For this review, use the dimensioned drawing (mm, ordinates from the lowest corner) and the shaded views. Round coordinates to 2 decimals unless told otherwise and drop trailing zeros. Order: outer loops, then holes, each group sorted by start corner. A loop starts at its lowest first (then second) coordinate and runs counter-clockwise, first axis right, second up. Notation, with made-up numbers: (-21, -10) - (-15, -10) arc R7 ccw to (-15, -6) - close; hole circle Ø9 at (37, 1). An arc over 180 degrees is marked (long way). Write item = value, one per line.
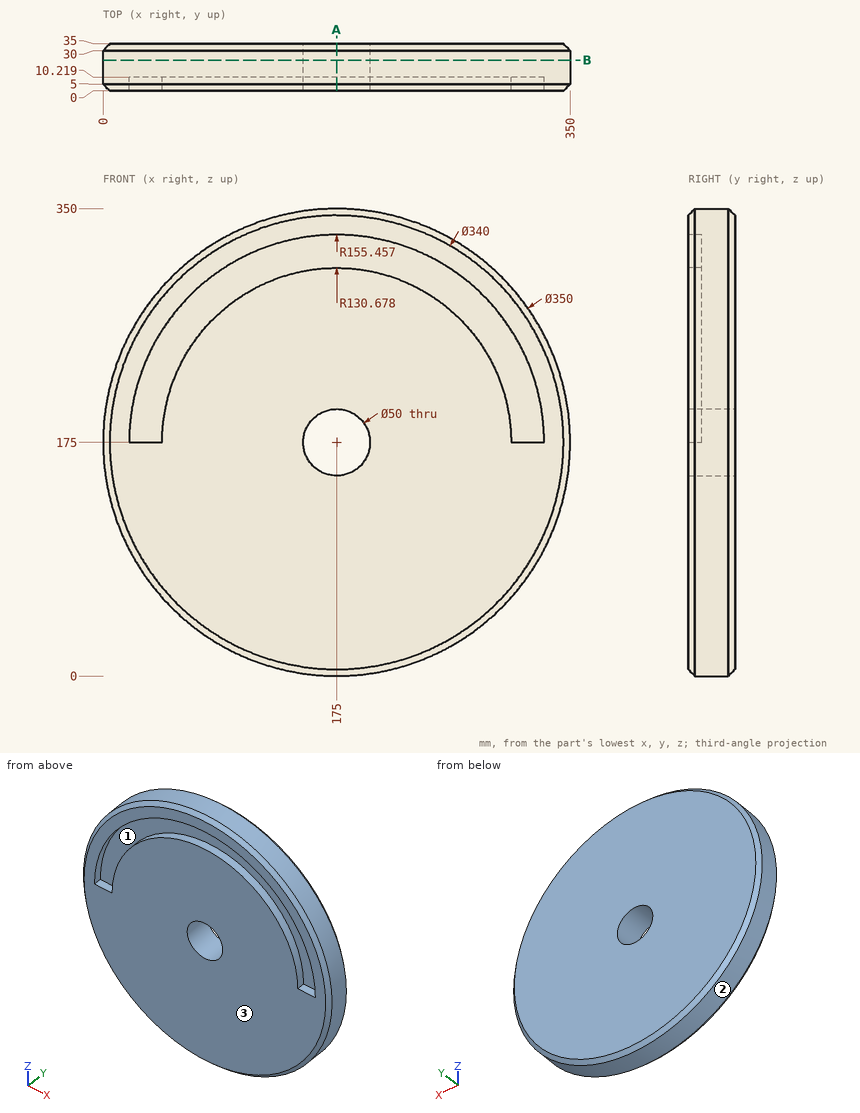
Item 1: Take a section at A-A, the plane x = 175. State the section outline as (y, z) points, and give its area (3 significant figures).
Data:
outline = (0, 5) - (5, 0) - (30, 0) - (35, 5) - (35, 150) - (0, 150) - close; (0, 200) - (35, 200) - (35, 345) - (30, 350) - (5, 350) - (0, 345) - (0, 330.46) - (10.22, 330.46) - (10.22, 305.68) - (0, 305.68) - close
area = 10,200 mm2
Item 2: For line 1 along Z through (x, y) = (175, 10); line 2 along Z through (x, y) = (175, 26); line 3 along Z through (x, y) = (197, 4.5) (1 decimal), list the stretches that pass through material, from the lowest coordinate up. Write a range as [from, to].
Data:
line_1 = [0, 150], [200, 305.68], [330.46, 350]
line_2 = [0, 150], [200, 350]
line_3 = [1.9, 163.1], [186.9, 303.8], [328.9, 348.1]
Item 3: Take a section at B-B, the plane y = 23. State the section outline as (x, z) points, and give its area (3 significant figures).
Data:
outline = circle Ø350 at (175, 175); hole circle Ø50 at (175, 175)
area = 94,200 mm2
Item 4: Insertion check: P1, Ø4, axis at x = 206, y = 14.5, coming from the -Z side; P2, Ø12, axis at y = 18.5, z = 163, coming from the -X side; P3, Ø3, axis at x = 101.5, y = 16, coming from the -Z side. Each pin has a flat end and moves straight along its axis. Give the tip position at first contact, or say it passes through.
Data:
P1 = 2.42
P2 = 0.1
P3 = 15.5
Item 5: The part is to be moulded in two halves that separate along X. For the marked faces 1, 2 and 3, say which applies: +X half, -X half, draft (parallel to the pull), parting line (faces both ways), or undercut.
Data:
face_1 = undercut
face_2 = parting line
face_3 = draft
